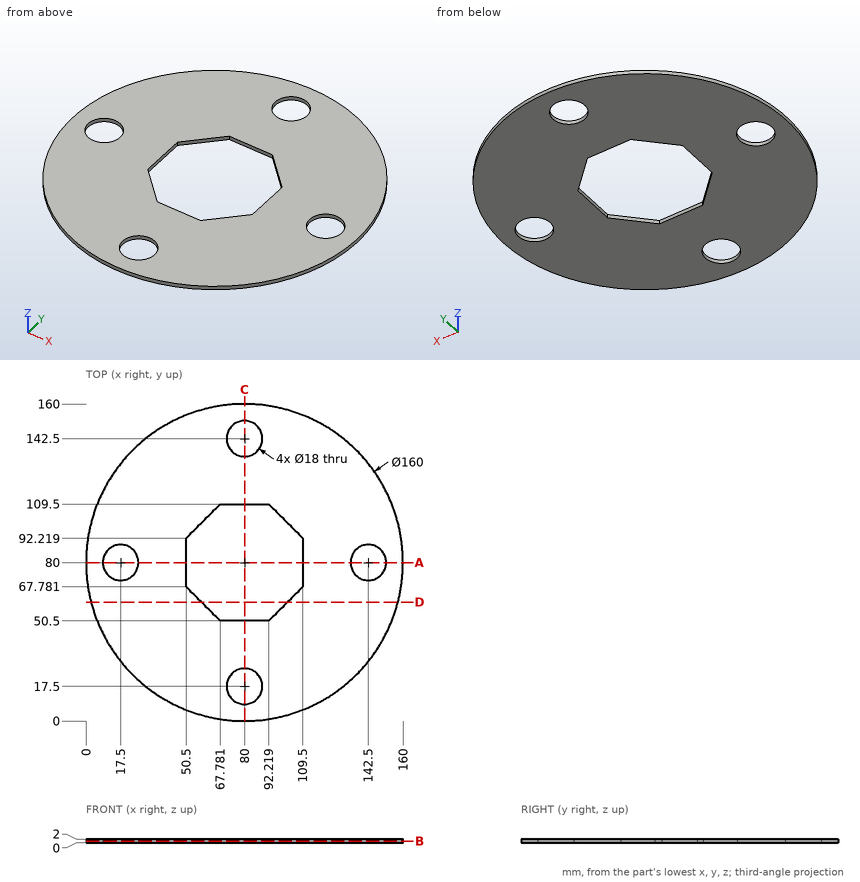
Design review of the part shown in the three views and the two pictorial views. Dimensions are in mm from the part's minimum x, y and z. Round coordinates to 2 decimals unless told otherwise and drop trailing zeros. Loops run counter-clockwise (first coordinate to the right, second up) from the corner with the lowest first, then second, coordinate; pieces in that order, holes last. Notation, with made-up numbers: M -12,-21.5 L 21,-21.5 A36 ccw 21,17.5 Z; hole C 11,67.5 d8. An arc over 180 degrees is marked long. Answer as a JSON object with one key per item and string values.
Item 1: Wall thickness on L1, parallel to Y at x = 80, z = 1.4; L2, parallel to Y at x = 82, z = 0.7 (1 decimal); L3, parallel to Y at x = 17.5, z = 0.7: over which ranges is each line inside the solid? List them lowest first. Write a range as from..to.
Answer sheet:
{"L1": "y = 0..8.5, 26.5..50.5, 109.5..133.5, 151.5..160", "L2": "y = 0..8.7, 26.3..50.5, 109.5..133.7, 151.3..160", "L3": "y = 30.06..71, 89..129.94"}
Item 2: Clearance check with flat-ended pins moving along their axes: P1, Ø0.6, axis at y = 83, z = 1.5, coming from the -X side; P2, Ø0.6, axis at y = 77, z = 1.5, coming from the +X side; P3, Ø1, axis at x = 85, z = 1, coming from the +Y side. State where each tip first meets the part, or that it passes through.
Answer sheet:
{"P1": "stops at x = 0.05", "P2": "stops at x = 159.95", "P3": "stops at y = 159.87"}
Item 3: We need section B-B on z = 0.95. Give the boundary of the cut face in (x, y), and give its area (3 significant figures).
Answer sheet:
{"outline": "C 80,80 d160; hole C 17.5,80 d18; hole M 50.5,67.78 L 67.78,50.5 L 92.22,50.5 L 109.5,67.78 L 109.5,92.22 L 92.22,109.5 L 67.78,109.5 L 50.5,92.22 Z; hole C 80,17.5 d18; hole C 80,142.5 d18; hole C 142.5,80 d18", "area": "16,200 mm^2"}
Item 4: We need section D-D on y = 60. Give the boundary of the cut face in (x, z).
Answer sheet:
{"outline": "M 2.54,0 L 58.28,0 L 58.28,2 L 2.54,2 Z; M 101.72,0 L 157.46,0 L 157.46,2 L 101.72,2 Z"}
Item 5: We need section A-A on y = 80. Give the boundary of the cut face in (x, z), and give its area (3 significant figures).
Answer sheet:
{"outline": "M 0,0 L 8.5,0 L 8.5,2 L 0,2 Z; M 26.5,0 L 50.5,0 L 50.5,2 L 26.5,2 Z; M 109.5,0 L 133.5,0 L 133.5,2 L 109.5,2 Z; M 151.5,0 L 160,0 L 160,2 L 151.5,2 Z", "area": "130 mm^2"}
